```python
from build123d import *

# Parameters (mm, degrees)
SKETCH1_R           = 77.003067154
SKETCH1_R_2         = 61.468535345
BOSS_EXTRUDE1_DEPTH = 10
BOSS_EXTRUDE2_DEPTH = 10
SKETCH3_W           = 26.477717066
SKETCH3_H           = 98.615222644
BOSS_EXTRUDE3_DEPTH = 10
SKETCH5_R           = 77.003067154
SKETCH5_R_2         = 61.468535345
BOSS_EXTRUDE4_DEPTH = 10
BOSS_EXTRUDE5_START = 10
BOSS_EXTRUDE5_DEPTH = 10
SKETCH8_W           = 26.477717066
SKETCH8_H           = 98.615222644
BOSS_EXTRUDE6_DEPTH = 10
SKETCH9_W           = 200
SKETCH9_H           = 520.453768192
BOSS_EXTRUDE7_DEPTH = 10


with BuildPart() as part:
    # Sketch1 → Boss-Extrude1 (new body)
    with BuildSketch(Plane(origin=(0, 0, 0), x_dir=(0, 0, -1), z_dir=(1, 0, 0))):
        Circle(SKETCH1_R)
        Circle(SKETCH1_R_2, mode=Mode.SUBTRACT)
    extrude(amount=BOSS_EXTRUDE1_DEPTH)

    # Sketch2 → Boss-Extrude2 (add)
    with BuildSketch(Plane(origin=(0, 0, 0), x_dir=(0, 0, -1), z_dir=(1, 0, 0))):
        with BuildLine():
            Line((-74.36042194, 20), (-233.957245684, 153.917635941))
            Line((-233.957245684, 153.917635941), (-260.43496275, 153.917635941))
            Line((-260.43496275, 153.917635941), (-77.003067154, 0))
            ThreePointArc((-77.003067154, 0), (-76.339547141, 10.086916944), (-74.36042194, 20))
        make_face()
    boss_extrude2 = extrude(amount=BOSS_EXTRUDE2_DEPTH)

    # Sketch3 → Boss-Extrude3 (add)
    with BuildSketch(Plane(origin=(0, 0, 0), x_dir=(0, 0, -1), z_dir=(1, 0, 0))):
        with Locations((-247.196104217, 203.225247263)):
            Rectangle(SKETCH3_W, SKETCH3_H)
    boss_extrude3 = extrude(amount=BOSS_EXTRUDE3_DEPTH)

    # Mirror2: Boss-Extrude2, Boss-Extrude3 across plane
    add(boss_extrude2.mirror(Plane.XY))
    add(boss_extrude3.mirror(Plane.XY))



with BuildPart() as body_2:
    # Sketch5 → Boss-Extrude4 (new body)
    with BuildSketch(Plane.ZY.offset(-200)):
        Circle(SKETCH5_R)
        with Locations(Location((0, 0, 0), (0, 0, 180))):
            Circle(SKETCH5_R_2, mode=Mode.SUBTRACT)
    extrude(amount=BOSS_EXTRUDE4_DEPTH)

    # Sketch7 → Boss-Extrude5 (add)
    with BuildSketch(Plane.ZY.offset(-200).offset(BOSS_EXTRUDE5_START)):
        with BuildLine():
            Line((-74.36042194, 20), (-233.957245684, 153.917635941))
            Line((-233.957245684, 153.917635941), (-260.43496275, 153.917635941))
            Line((-260.43496275, 153.917635941), (-77.003067154, 0))
            ThreePointArc((-77.003067154, 0), (-76.339547141, 10.086916944), (-74.36042194, 20))
        make_face()
    boss_extrude5 = extrude(amount=-BOSS_EXTRUDE5_DEPTH)

    # Sketch8 → Boss-Extrude6 (add)
    with BuildSketch(Plane.ZY.offset(-200)):
        with Locations((-247.196104217, 203.225247263)):
            Rectangle(SKETCH8_W, SKETCH8_H)
    boss_extrude6 = extrude(amount=BOSS_EXTRUDE6_DEPTH)

    # Mirror5: Boss-Extrude5 across plane
    add(boss_extrude5.mirror(Plane.XY))

    # Mirror6: Boss-Extrude6 across plane
    add(boss_extrude6.mirror(Plane.XY))


with BuildPart() as part_1:
    add(part.part)

    add(body_2.part)  # Boss-Extrude7 merges body 2
    # Sketch9 → Boss-Extrude7 (add)
    with BuildSketch(Plane(origin=(0, 250, 0), x_dir=(1, 0, 0), z_dir=(0, 1, 0))):
        with Locations((100, 0.208078654)):
            Rectangle(SKETCH9_W, SKETCH9_H)
    extrude(amount=BOSS_EXTRUDE7_DEPTH)


solid = part_1.part
```
Read the model definition and answer for the solid it produces. Units are mm, in the model's axes. A direction names the side the tool comes from. Coordinates: 2 decimals unless noted, no trailing zeros. Loops run counter-clockwise (first coordinate to the right, second up) from the corner with the lowest first, then second, coordinate; pieces in that order, holes last. Notation, with made-up numbers: (62, 42.25) - (68, 42.25) arc R29 cw to (68, 63.25) - close; hole circle Ø4 at (-8.5, 50). An arc over 180 degrees is marked (long way). Answer in a Markdown table with one row per item.
1. Straight lines are drawn through the part: line 1 (Y direction, x = 7, z = 0); line 2 (Y direction, x = 28, z = 97.5). For each, find the intervals that lie inside material, in ascending order.
Conclusion:
| item | result |
|---|---|
| line 1 | y = -77 to -61.47, 61.47 to 77, 250 to 260 |
| line 2 | y = 250 to 260 |
2. Determine the mould class of faces 3 (the face through (10, 76, -1)), 4 (the face through (195.07, 76.99, 1.41)), 5 (the face through (4.93, -76.984, 1.693)) for opening direction Z: +Z half, -Z half, draft (parallel to the pull), parting line (faces both ways), or undercut.
Conclusion:
| item | result |
|---|---|
| face 3 | draft |
| face 4 | undercut |
| face 5 | parting line |
3. Find section C-C, the plane z = -165. Write down the section's boundary in (x, y).
Conclusion:
| item | result |
|---|---|
| outline | (0, 73.84) - (10, 73.84) - (10, 96.06) - (0, 96.06) - close; (0, 250) - (200, 250) - (200, 260) - (0, 260) - close; (190, 73.84) - (200, 73.84) - (200, 96.06) - (190, 96.06) - close |
4. Which of the six approach directions +Z, -Z, +X, -X, +Y, -Y give full straight-line access (tool end or side, diameter ignored) to faces 1 (the face through (99, 260, -4)), 2 (the face through (5, 201, -233.957))?
Conclusion:
| item | result |
|---|---|
| face 1 | +Z, -Z, +X, -X, +Y |
| face 2 | +X, -X |
5. Find section D-D, the plane x = 93. Write down the section's boundary in (y, z), then the cut area to 3 significant figures.
Conclusion:
| item | result |
|---|---|
| outline | (250, -260.43) - (260, -260.43) - (260, 260.02) - (250, 260.02) - close |
| area | 5,200 mm² |
6. Given pin 1 (11 mm diameter, centred on x = 63.5, y = 255.5, fed in from +Z); pin 2 (0.5 mm diameter, centred on x = 196.5, z = 260.5, fed in from +Y); pin 3 (10 mm diameter, centred on x = 173, z = 113.5, fed in from -Y), each flat-ended and moving along its own axis, determine where each tip first touches the part or whether it passes through.
Conclusion:
| item | result |
|---|---|
| pin 1 | stops at z = 260.02 |
| pin 2 | stops at y = 252.53 |
| pin 3 | stops at y = 250 |
7. Find section B-B, the plane z = 0. Write down the section's boundary in (x, y).
Conclusion:
| item | result |
|---|---|
| outline | (0, -77) - (10, -77) - (10, -61.47) - (0, -61.47) - close; (0, 61.47) - (10, 61.47) - (10, 77) - (0, 77) - close; (0, 250) - (200, 250) - (200, 260) - (0, 260) - close; (190, -77) - (200, -77) - (200, -61.47) - (190, -61.47) - close; (190, 61.47) - (200, 61.47) - (200, 77) - (190, 77) - close |
8. Find section A-A, the plane y = 179.5. Write down the section's boundary in (x, z).
Conclusion:
| item | result |
|---|---|
| outline | (0, -260.43) - (10, -260.43) - (10, -233.96) - (0, -233.96) - close; (0, 233.96) - (10, 233.96) - (10, 260.43) - (0, 260.43) - close; (190, -260.43) - (200, -260.43) - (200, -233.96) - (190, -233.96) - close; (190, 233.96) - (200, 233.96) - (200, 260.43) - (190, 260.43) - close |
